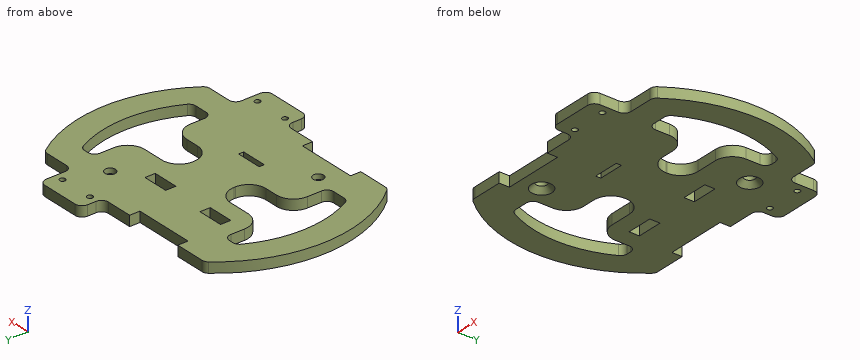
```python
from build123d import *

# Parameters (mm, degrees)
ESBO_O1_R                = 3.05
ESBO_O1_W                = 15
ESBO_O1_H                = 3
ESBO_O1_R_2              = 1.6
ESBO_O1_H_2              = 6
RESSALTO_EXTRUS_O1_DEPTH = 6
CHANFRO1_SIZE            = 3
FILETE1_R                = 4
FILETE2_R                = 10
FILETE3_R                = 10


with BuildPart() as part:
    # Esboço1 → Ressalto-extrusão1 (new body)
    with BuildSketch(Plane.XY):
        with BuildLine():
            Line((14.471901241, -53.5), (14.471901241, -66.5))
            Line((14.471901241, -66.5), (44.471901241, -66.5))
            Line((44.471901241, -66.5), (44.471901241, -47.5))
            Line((44.471901241, -47.5), (64.371965948, -47.5))
            ThreePointArc((64.371965948, -47.5), (80, 0), (64.371965948, 47.5))
            Line((64.371965948, 47.5), (44.471901241, 47.5))
            Line((44.471901241, 47.5), (44.471901241, 66.5))
            Line((44.471901241, 66.5), (14.471901241, 66.5))
            Line((14.471901241, 66.5), (14.471901241, 53.5))
            Line((14.471901241, 53.5), (-5.003543323, 53.5))
            Line((-5.003543323, 53.5), (-5.003543323, 47.5))
            Line((-5.003543323, 47.5), (-40.003543323, 47.5))
            Line((-40.003543323, 47.5), (-40.003543323, 53.5))
            Line((-40.003543323, 53.5), (-59.478987886, 53.5))
            ThreePointArc((-59.478987886, 53.5), (-80, 0), (-59.478987886, -53.5))
            Line((-59.478987886, -53.5), (-40.003543323, -53.5))
            Line((-40.003543323, -53.5), (-40.003543323, -47.5))
            Line((-40.003543323, -47.5), (-5.003543323, -47.5))
            Line((-5.003543323, -47.5), (-5.003543323, -53.5))
            Line((-5.003543323, -53.5), (14.471901241, -53.5))
        make_face()
        with BuildLine():
            Line((-56.291651246, 32.5), (-47.55, 32.5))
            Line((-47.55, 32.5), (-47.55, 10.5))
            Line((-47.55, 10.5), (-15, 10.5))
            Line((-15, 10.5), (-15, -10.2))
            Line((-15, -10.2), (-42.5, -10.2))
            Line((-42.5, -10.2), (-42.5, -32.5))
            Line((-42.5, -32.5), (-56.291651246, -32.5))
            ThreePointArc((-56.291651246, -32.5), (-65, 0), (-56.291651246, 32.5))
        make_face(mode=Mode.SUBTRACT)
        with BuildLine():
            Line((47.55, 32.5), (56.291651246, 32.5))
            ThreePointArc((56.291651246, 32.5), (65, 0), (56.291651246, -32.5))
            Line((56.291651246, -32.5), (42.5, -32.5))
            Line((42.5, -32.5), (42.5, -10.2))
            Line((42.5, -10.2), (15, -10.2))
            Line((15, -10.2), (15, 10.5))
            Line((15, 10.5), (47.55, 10.5))
            Line((47.55, 10.5), (47.55, 32.5))
        make_face(mode=Mode.SUBTRACT)
        with Locations((-31.783703802, -35.29937921)):
            Circle(ESBO_O1_R, mode=Mode.SUBTRACT)
        with Locations((0, -21.7)):
            Rectangle(ESBO_O1_W, ESBO_O1_H, mode=Mode.SUBTRACT)
        with Locations((19.471901241, -57)):
            Circle(ESBO_O1_R_2, mode=Mode.SUBTRACT)
        with Locations((39.471901241, -57)):
            Circle(ESBO_O1_R_2, mode=Mode.SUBTRACT)
        with Locations((-30.05, 23.5)):
            Rectangle(ESBO_O1_W, ESBO_O1_H_2, mode=Mode.SUBTRACT)
        with Locations((9.95, 23.5)):
            Rectangle(ESBO_O1_W, ESBO_O1_H_2, mode=Mode.SUBTRACT)
        with Locations((31.783703802, 35.29937921)):
            Circle(ESBO_O1_R, mode=Mode.SUBTRACT)
        with Locations((19.471901241, 57)):
            Circle(ESBO_O1_R_2, mode=Mode.SUBTRACT)
        with Locations((39.471901241, 57)):
            Circle(ESBO_O1_R_2, mode=Mode.SUBTRACT)
    extrude(amount=RESSALTO_EXTRUS_O1_DEPTH)

    # Chanfro1
    chanfro1_edges = [part.edges().sort_by_distance(p)[0] for p in [
        (-34.833703802, -35.29937921, 0),
        (28.733703802, 35.29937921, 0),
    ]]
    chamfer(chanfro1_edges, length=CHANFRO1_SIZE)

    # Filete1
    filete1_edges = [part.edges().sort_by_distance(p)[0] for p in [
        (-42.5, -32.5, 3),
        (-47.55, 32.5, 3),
        (-56.291651246, 32.5, 3),
        (-56.291651246, -32.5, 3),
        (56.291651246, 32.5, 3),
        (47.55, 32.5, 3),
        (42.5, -32.5, 3),
        (56.291651246, -32.5, 3),
        (44.471901241, -47.5, 3),
        (44.471901241, -66.5, 3),
        (14.471901241, -66.5, 3),
        (14.471901241, -53.5, 3),
        (-59.478987886, -53.5, 3),
        (-59.478987886, 53.5, 3),
        (14.471901241, 53.5, 3),
        (14.471901241, 66.5, 3),
        (44.471901241, 66.5, 3),
        (44.471901241, 47.5, 3),
        (64.371965948, 47.5, 3),
        (64.371965948, -47.5, 3),
    ]]
    fillet(filete1_edges, radius=FILETE1_R)

    # Filete2
    filete2_edges = [part.edges().sort_by_distance(p)[0] for p in [
        (-15, -10.2, 3),
        (-15, 10.5, 3),
        (15, 10.5, 3),
        (15, -10.2, 3),
    ]]
    fillet(filete2_edges, radius=FILETE2_R)

    # Filete3
    filete3_edges = [part.edges().sort_by_distance(p)[0] for p in [
        (-42.5, -10.2, 3),
        (-47.55, 10.5, 3),
        (47.55, 10.5, 3),
        (42.5, -10.2, 3),
    ]]
    fillet(filete3_edges, radius=FILETE3_R)


solid = part.part
```
Input: part model. Units: mm. Frame: model coordinates. Round coordinates to 2 decimals unless told otherwise and drop trailing zeros. Loops run counter-clockwise (first coordinate to the right, second up) from the corner with the lowest first, then second, coordinate; pieces in that order, holes last. Notation, with made-up numbers: (49, 67) -> (72, 67) arc R18 ccw to (72, 100) -> close; hole circle Ø5 at (80.5, 36). An arc over 180 degrees is marked (long way). Use one line per item in the form item = value. Start each with the question number.
Item 1: Section query D-D on z = 4.8. Count the separate pieces of the cut face and the enclosed holes in it, then the cut area to 3 significant figures.
Item 2: Section query C-C on x = -44.5. Return the cut outline in (y, z).
Item 3: Section query A-A on x = -2.5. Return the cut outline in (y, z).
Item 4: Material intervals for L1, parallel to Y at x = 26, z = 1.85; L2, parallel to X at y = 3, z = 3.2; L3, parallel to X at y = -28, z = 1.2, sorted ascending. Write a range as from..to.
Item 5: Contact query for flat-ended pins moving along their axis: pin 1 Ø3 at (y, z) = (-49.5, 1.5) entering from +X; pin 2 Ø0.7 at (x, z) = (53, 3) entering from -Y; pin 3 Ø3 at (y, z) = (50.5, 2) entering from +X; pin 4 Ø4 at (x, y) = (-17, 50) entering from +Z. Output: stop coordinate, or through.
Item 6: Section query B-B on y = -12. Return the cut outline in (x, z), then the cut area to 3 significant figures.
Ans:
q1.separate_pieces = 1
q1.enclosed_holes = 11
q1.area = 12,100 mm^2
q2.outline = (-53.5, 0) -> (-31.96, 0) -> (-31.96, 6) -> (-53.5, 6) -> close; (13.31, 0) -> (53.5, 0) -> (53.5, 6) -> (13.31, 6) -> close
q3.outline = (-53.5, 0) -> (-23.2, 0) -> (-23.2, 6) -> (-53.5, 6) -> close; (-20.2, 0) -> (53.5, 0) -> (53.5, 6) -> (-20.2, 6) -> close
q4.L1 = -66.5..-10.2, 10.5..66.5
q4.L2 = -79.94..-64.93, -15.32..15.32, 64.93..79.94
q4.L3 = -74.94..-58.66, -42.5..42.5, 58.66..74.94
q5.pin_1 = 46.54
q5.pin_2 = -47.5
q5.pin_3 = 45.35
q5.pin_4 = through
q6.outline = (-79.09, 0) -> (-63.88, 0) -> (-63.88, 6) -> (-79.09, 6) -> close; (-38.22, 0) -> (38.22, 0) -> (38.22, 6) -> (-38.22, 6) -> close; (63.88, 0) -> (79.09, 0) -> (79.09, 6) -> (63.88, 6) -> close
q6.area = 641 mm^2
